For this review, take the finished solid that the model builds, in its own axes (mm). Face numbers are marked on the shaded views. A direction names the side the tool comes from. Coordinates: 2 decimals unless noted, no trailing zeros. Loops run counter-clockwise (first coordinate to the right, second up) from the corner with the lowest first, then second, coordinate; pieces in that order, holes last. Notation, with made-up numbers: M -3,-1 L 43,-1 A11 cw 43,11 Z; hole C 22,-30 d8. An arc over 180 degrees is marked long. Write item = value, one per line.
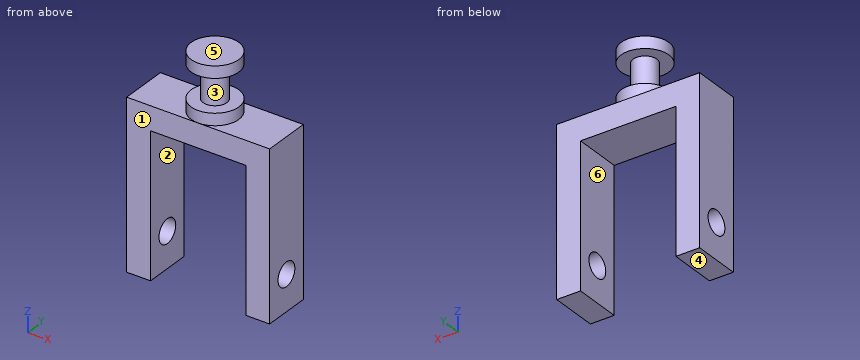
from build123d import *

# Parameters (mm, degrees)
SKETCH1_R               = 25.4
BOSS_EXTRUDE1_DEPTH     = 12.7
SKETCH2_R               = 12.7
BOSS_EXTRUDE2_DEPTH     = 35.4
SKETCH3_R               = 25.4
BOSS_EXTRUDE3_DEPTH     = 12.7
SKETCH4_W               = 152.4
SKETCH4_H               = 50.8
BOSS_EXTRUDE4_DEPTH     = 25.4
SKETCH5_W               = 25.4
SKETCH5_H               = 50.8
BOSS_EXTRUDE5_DEPTH     = 152.4
CUT_EXTRUDE1_DEPTH      = 285.254955981
CUT_EXTRUDE1_DEPTH_BACK = 285.254955981
SKETCH6_R               = 12.7


with BuildPart() as part:
    # Sketch1 → Boss-Extrude1 (new body)
    with BuildSketch(Plane.XY):
        Circle(SKETCH1_R)
    extrude(amount=-BOSS_EXTRUDE1_DEPTH)

    # Sketch2 → Boss-Extrude2 (add)
    with BuildSketch(Plane(origin=(0, 0, -12.7), x_dir=(-1, 0, 0), z_dir=(0, 0, -1))):
        Circle(SKETCH2_R)
    extrude(amount=BOSS_EXTRUDE2_DEPTH)

    # Sketch3 → Boss-Extrude3 (add)
    with BuildSketch(Plane(origin=(0, 0, -48.1), x_dir=(-1, 0, 0), z_dir=(0, 0, -1))):
        with Locations(Location((0, 0, 0), (0, 0, 180))):
            Circle(SKETCH3_R)
    extrude(amount=BOSS_EXTRUDE3_DEPTH)

    # Sketch4 → Boss-Extrude4 (add)
    with BuildSketch(Plane(origin=(0, 0, -60.8), x_dir=(-1, 0, 0), z_dir=(0, 0, -1))):
        Rectangle(SKETCH4_W, SKETCH4_H)
    extrude(amount=BOSS_EXTRUDE4_DEPTH)

    # Sketch5 → Boss-Extrude5 (add)
    with BuildSketch(Plane(origin=(0, 0, -86.2), x_dir=(-1, 0, 0), z_dir=(0, 0, -1))):
        with Locations((-63.5, 0)):
            Rectangle(SKETCH5_W, SKETCH5_H)
        with Locations((63.5, 0)):
            Rectangle(SKETCH5_W, SKETCH5_H)
    extrude(amount=BOSS_EXTRUDE5_DEPTH)

    # Sketch6 → Cut-Extrude1 (cut, two sides: drawn at the far end of the back side and taken through both)
    with BuildSketch(Plane.ZY.offset(76.2).offset(-CUT_EXTRUDE1_DEPTH_BACK)):
        with Locations((-200.5, 0)):
            Circle(SKETCH6_R)
    extrude(amount=CUT_EXTRUDE1_DEPTH + CUT_EXTRUDE1_DEPTH_BACK, mode=Mode.SUBTRACT)


solid = part.part
Q1. Machinability: for the marked faces 1 and 2, which of the approach directions +Z, -Z, +X, -X, +Y, -Y give a long, thin tool a straight path to every point of the face, cutting with its end or side? Answer none if there is none.
Solved:
face_1 = +Z, -Z, +X, -X, -Y
face_2 = -Z, +Y, -Y
Q2. Add section D-D (x = -61.5). Write out the cut boundary in (y, z), and give its area (3 significant figures).
Solved:
outline = M -25.4,-238.6 L 25.4,-238.6 L 25.4,-60.8 L -25.4,-60.8 Z; hole C 0,-200.5 d25.4
area = 8,530 mm²
Q3. Add section A-A (z = -200.5). Write out the cut boundary in (x, y), and give its area (3 significant figures).
Solved:
outline = M -76.2,-25.4 L -50.8,-25.4 L -50.8,-12.7 L -76.2,-12.7 Z; M -76.2,12.7 L -50.8,12.7 L -50.8,25.4 L -76.2,25.4 Z; M 50.8,-25.4 L 76.2,-25.4 L 76.2,-12.7 L 50.8,-12.7 Z; M 50.8,12.7 L 76.2,12.7 L 76.2,25.4 L 50.8,25.4 Z
area = 1,290 mm²
Q4. Add section B-B (y = 0). Write out the cut boundary in (x, z), and give its area (3 significant figures).
Solved:
outline = M -76.2,-238.6 L -50.8,-238.6 L -50.8,-213.2 L -76.2,-213.2 Z; M -76.2,-187.8 L -50.8,-187.8 L -50.8,-86.2 L 50.8,-86.2 L 50.8,-187.8 L 76.2,-187.8 L 76.2,-60.8 L 25.4,-60.8 L 25.4,-48.1 L 12.7,-48.1 L 12.7,-12.7 L 25.4,-12.7 L 25.4,0 L -25.4,0 L -25.4,-12.7 L -12.7,-12.7 L -12.7,-48.1 L -25.4,-48.1 L -25.4,-60.8 L -76.2,-60.8 Z; M 50.8,-238.6 L 76.2,-238.6 L 76.2,-213.2 L 50.8,-213.2 Z
area = 12,500 mm²
Q5. Add section C-C (z = -159). Write out the cut boundary in (x, y), and give its area (3 significant figures).
Solved:
outline = M -76.2,-25.4 L -50.8,-25.4 L -50.8,25.4 L -76.2,25.4 Z; M 50.8,-25.4 L 76.2,-25.4 L 76.2,25.4 L 50.8,25.4 Z
area = 2,580 mm²
Q6. For pin 1 Ø12 at (x, y) = (-26.5, -2) entering from -Z; pin 2 Ø6 at (x, y) = (32, -6) entering from +Z; pin 3 Ø4 at (y, z) = (-10, -55.5) entering from +X; pin 4 Ø20.5 at (y, z) = (0, -200.5) entering from +X, all flat-tipped, find the tip position at first contact; note any pin that passes through.
Solved:
pin_1 = -86.2
pin_2 = -60.8
pin_3 = 24.11
pin_4 = through
Q7. Draft analysis for pull direction Z (two halves, no side actions). For the marked faces 3, 4, 5 and 6, state which applies: +Z half, -Z half, draft (parallel to the pull), parting line (faces both ways), or undercut.
Solved:
face_3 = undercut
face_4 = -Z half
face_5 = +Z half
face_6 = draft
Q8. For line 1 along X through (y, z) = (-21.5, -180.5); line 2 along Y through (x, z) = (64, -200); line 3 along Z through (x, y) = (68.5, 0), list the stretches that pass through material, from the lowest coordinate up.
Solved:
line_1 = -76.2 to -50.8, 50.8 to 76.2
line_2 = -25.4 to -12.69, 12.69 to 25.4
line_3 = -238.6 to -213.2, -187.8 to -60.8
